Source: three-view drawing plus pictorial views. Frame: mm from the lowest corner of the part. Give positions to 0.01 mm unless a question says otherwise; leave off trailing zeros. Loops run counter-clockwise (first coordinate to the right, second up) from the corner with the lowest first, then second, coordinate; pieces in that order, holes last. Notation, with made-up numbers: (45.25, 64) -> (86.25, 64) arc R25 cw to (86.25, 81) -> close; hole circle Ø11 at (-32.75, 78.5). An arc over 180 degrees is marked (long way). Put each result on its own line as item: value.
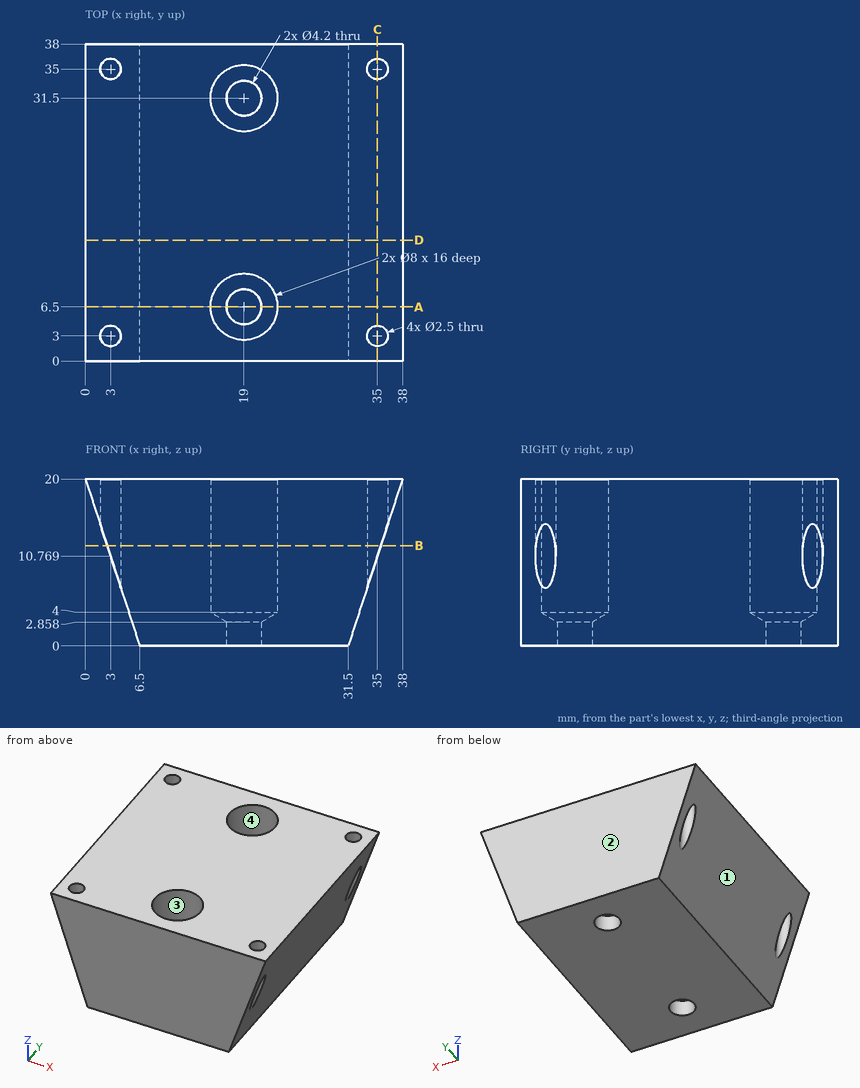
(1) Line query: probe 1 along Y at (x, z) = (35, 12.75); probe 2 along Y at (x, z) = (19, 12); probe 3 along X at (y, z) = (6.5, 1) (1 decimal). Output: solid intervals per line, ascending. Write a range as from..to.
Calculated:
probe 1: y = 0..1.75, 4.25..33.75, 36.25..38
probe 2: y = 0..2.5, 10.5..27.5, 35.5..38
probe 3: x = 6.2..16.9, 21.1..31.8
(2) Section A-A on y = 6.5. Return loops of the section in (x, z), then the cut area to 3 significant figures.
Calculated:
outline: (0, 20) -> (6.5, 0) -> (16.9, 0) -> (16.9, 2.86) -> (15, 4) -> (15, 20) -> close; (21.1, 0) -> (31.5, 0) -> (38, 20) -> (23, 20) -> (23, 4) -> (21.1, 2.86) -> close
area: 483 mm²
(3) Section B-B on z = 12. Give the number of separate pieces and of enclosed holes in the cut face, then the cut area to 3 significant figures.
Calculated:
separate pieces: 1
enclosed holes: 2
area: 1,130 mm²
(4) Draft query along Y for the marked faces 1, 2, 3 and 4. Return one class per face: released by +Y, released by -Y, zero draft, split by the parting line, or undercut.
Calculated:
face 1: zero draft
face 2: released by +Y
face 3: undercut
face 4: undercut
(5) Section C-C on x = 35. Return loops of the section in (y, z).
Calculated:
outline: (0, 10.77) -> (1.75, 10.77) -> (1.75, 20) -> (0, 20) -> close; (4.25, 10.77) -> (33.75, 10.77) -> (33.75, 20) -> (4.25, 20) -> close; (36.25, 10.77) -> (38, 10.77) -> (38, 20) -> (36.25, 20) -> close
(6) Section D-D on y = 14.5. Return loops of the section in (x, z), then the cut area to 3 significant figures.
Calculated:
outline: (0, 20) -> (6.5, 0) -> (31.5, 0) -> (38, 20) -> close
area: 630 mm²
(7) First-contact query: P1, Ø1.5, axis at y = 10, z = 9, coming from the -X side; P2, Ø12, axis at y = 30, z = 3.5, coming from the +X side; P3, Ø1.5, axis at y = 14.5, z = 13.5, coming from the -X side. Flat tips, straight axial feed; report the tip coordinate or a pass-through.
Calculated:
P1: stops at x = 3.33
P2: stops at x = 34.59
P3: stops at x = 1.87
